Geometry check sheet. Reference: the model listing, model coordinates, mm. A direction names the side the tool comes from. Round coordinates to 2 decimals unless told otherwise and drop trailing zeros. Order: outer loops, then holes, each group sorted by start corner. A loop starts at its lowest first (then second) coordinate and runs counter-clockwise, first axis right, second up. Notation, with made-up numbers: (49, 17) - (75, 17) arc R25 ccw to (75, 47) - close; hole circle Ø1 at (47.5, 38). An arc over 180 degrees is marked (long way). One line per question, with ' | ' between items. Start each with the question number.
Q1. Sectioned sample at D-D, the plane y = 21.5. Enter the section's corners in (x, z), then the cut area to 3 significant figures.
Q2. Material ranges on line 1 along Y through (x, z) = (-5.5, 21.25); line 2 along X through (y, z) = (6.5, 5.25); line 3 along Z through (x, y) = (-13.5, 2.75), recorded low to high.
Q3. Gauge pin test, flat ends, axial feed: P1, Ø4.5, axis at x = -16, y = 4.5, coming from the +Z side; P2, Ø1.5, axis at x = -13, z = 12, coming from the +Y side; P3, Ø3, axis at y = 10.5, z = 13, coming from the -X side. Record the tip position at first contact, or that the pin passes through.
Q4. Sectioned sample at B-B, the plane z = 5. Enter the section's corners in (x, y).
Q5. Mould release check, pull along Y, two halves, no side actions. Record for faces 3 (the face through (-8.46, 1.12, 14.79)), 4 (the face through (-23.226, 6.309, 12.572)), 5 (the face through (-23.25, 23.72, 12.57)), 6 (the face through (-3, 15, 28)): +Y half, -Y half, draft (parallel to the pull), parting line (faces both ways), or undercut.
Q6. Tool access check on faces 1 (the face through (-20.039, 26.875, 12.572)), 2 (the face through (-13, 26, 25.5)). Record the directions out of +Z, -Z, +X, -X, +Y, -Y that give a thin tool (end or side, any length) a straight path to the whole face; none if there is none.
Q7. Sectioned sample at C-C, the plane x = -19. Enter the section's corners in (y, z), then the cut area to 3 significant figures.
Q8. Sectioned sample at A-A, the plane x = -9. Enter the section's corners in (y, z).
```python
from build123d import *

# Parameters (mm, degrees)
F1_DEPTH = 30
F3_DEPTH = 40


with BuildPart() as f1:
    # F0 (on Top) → F1 (new body)
    with BuildSketch(Plane.XY):
        with BuildLine():
            Line((-16.694256, 2.211744), (0, 0))
            Line((0, 0), (10.5, 0))
            Line((10.5, 0), (10.5, 30))
            Line((10.5, 30), (0, 30))
            Line((0, 30), (-16.694256, 27.788256))
            ThreePointArc((-16.694256, 27.788256), (-20.084053, 26.855902), (-23.096234, 25.042957))
            ThreePointArc((-23.096234, 25.042957), (-23.239598, 23.707125), (-21.903766, 23.563762))
            ThreePointArc((-21.903766, 23.563762), (-10.253497, 24.923241), (-4, 15))
            ThreePointArc((-4, 15), (-10.253497, 5.076759), (-21.903766, 6.436238))
            ThreePointArc((-21.903766, 6.436238), (-23.239598, 6.292875), (-23.096234, 4.957043))
            ThreePointArc((-23.096234, 4.957043), (-20.084053, 3.144098), (-16.694256, 2.211744))
        make_face()
    extrude(amount=F1_DEPTH)

    # F2 (on face) → F3 (cut)
    with BuildSketch(Plane.XZ):
        Polygon((0, 35.99402), (-26.560755, 35.99402), (-26.560755, 25.5), (-5.5, 25.5), (-1, 30), (0, 30), align=None)
    extrude(amount=-F3_DEPTH, mode=Mode.SUBTRACT)


solid = f1.part
```
Determined:
1) outline: (-6.13, 0) - (10.5, 0) - (10.5, 30) - (-1, 30) - (-5.5, 25.5) - (-6.13, 25.5) - close | area: 486 mm2
2) line 1: y = 0.73 to 9.45, 20.55 to 29.27 | line 2: x = -23.01 to -21.99, -8.02 to 10.5 | line 3: z = 0 to 25.5
3) P1: stops at z = 25.5 | P2: stops at y = 28.38 | P3: stops at x = -5.78
4) outline: (-23.1, 4.96) arc R12.9 ccw to (-16.69, 2.21) - (0, 0) - (10.5, 0) - (10.5, 30) - (0, 30) - (-16.69, 27.79) arc R12.9 ccw to (-23.1, 25.04) arc R0.95 ccw to (-21.9, 23.56) arc R11 cw (long way) to (-21.9, 6.44) arc R0.95 ccw to start
5) face 3: -Y half | face 4: undercut | face 5: undercut | face 6: draft
6) face 1: +Z, -Z, -X, +Y | face 2: +Z, -X, +Y, -Y
7) outline: (2.74, 0) - (4.75, 0) - (4.75, 25.5) - (2.74, 25.5) - close; (25.25, 0) - (27.26, 0) - (27.26, 25.5) - (25.25, 25.5) - close | area: 103 mm2
8) outline: (1.19, 0) - (5.78, 0) - (5.78, 25.5) - (1.19, 25.5) - close; (24.22, 0) - (28.81, 0) - (28.81, 25.5) - (24.22, 25.5) - close
